from build123d import *

# Parameters (mm, degrees)
F1_DEPTH = 38.1


with BuildPart() as f1:
    # F0 (on Right) → F1 (new body, symmetric)
    with BuildSketch(Plane.YZ):
        with BuildLine():
            ThreePointArc((-6.350009, 50.8), (10.388841, 10.388841), (50.8, -6.350009))
            Line((50.8, -6.350009), (353.615227, -6.350009))
            ThreePointArc((353.615227, -6.350009), (404.926872, 25.635765), (398.802211, 85.789428))
            Line((398.802211, 85.789428), (95.986983, 476.859172))
            ThreePointArc((95.986983, 476.859172), (32.310989, 495.946356), (-6.350009, 441.869744))
            Line((-6.350009, 441.869744), (-6.350009, 50.8))
        make_face()
        with BuildLine():
            Line((0, 50.8), (0, 441.869744))
            ThreePointArc((0, 441.869744), (34.365327, 489.937836), (90.966201, 472.971453))
            Line((90.966201, 472.971453), (393.781428, 81.901709))
            ThreePointArc((393.781428, 81.901709), (399.22557, 28.431795), (353.615227, 0))
            Line((353.615227, 0), (50.8, 0))
            ThreePointArc((50.8, 0), (14.878976, 14.878976), (0, 50.8))
        make_face(mode=Mode.SUBTRACT)
    extrude(amount=F1_DEPTH, both=True)


solid = f1.part
For this review, take the finished solid that the model builds, in its own axes (mm). A direction names the side the tool comes from. Round coordinates to 2 decimals unless told otherwise and drop trailing zeros. Loops run counter-clockwise (first coordinate to the right, second up) from the corner with the lowest first, then second, coordinate; pieces in that order, holes last. Notation, with made-up numbers: (37.25, 83.5) - (42.25, 83.5) arc R15 ccw to (42.25, 93.5) - close; hole circle Ø10 at (-24.75, 61). An arc over 180 degrees is marked (long way). Use one line per item in the form item = value.
Item 1: Consider section B-B on x = -13.5. Write out the cut boundary in (y, z).
Answers:
outline = (-6.35, 50.8) arc R57.15 ccw to (50.8, -6.35) - (353.62, -6.35) arc R57.15 ccw to (398.8, 85.79) - (95.99, 476.86) arc R57.15 ccw to (-6.35, 441.87) - close; hole (0, 50.8) arc R50.8 ccw to (50.8, 0) - (353.62, 0) arc R50.8 ccw to (393.78, 81.9) - (90.97, 472.97) arc R50.8 ccw to (0, 441.87) - close
Item 2: Mouldability with a two-part tool opening along Y and no side actions: class faces 1 (the cylindrical face through (0.533, 33.532, 489.645)), 2 (the cylindrical face through (0.53, 33.25, 496.26)), 3 (the flat face through (38.1, 186, 360)) as +Y half, -Y half, draft (parallel to the pull), parting line (faces both ways), or undercut.
Answers:
face_1 = undercut
face_2 = parting line
face_3 = draft
Item 3: Consider section C-C on z = 343.5. Write out the cut boundary in (x, y).
Answers:
outline = (-38.1, -6.35) - (38.1, -6.35) - (38.1, 0) - (-38.1, 0) - close; (-38.1, 191.22) - (38.1, 191.22) - (38.1, 199.25) - (-38.1, 199.25) - close
Item 4: For line 1 (Y direction, x = 10.5, z = 329.5); line 2 (Y direction, x = 16, z = 18); line 3 (Z direction, x = -12, y = 268), list the stretches that pass through material, from the lowest coordinate up.
Answers:
line_1 = -6.35 to 0, 202.06 to 210.09
line_2 = 4 to 12.01, 392.41 to 400.42
line_3 = -6.35 to 0, 244.34 to 254.71
Item 5: Consider section A-A on y = 164. Write out the cut boundary in (x, z), then the cut area to 3 significant figures.
Answers:
outline = (-38.1, -6.35) - (38.1, -6.35) - (38.1, 0) - (-38.1, 0) - close; (-38.1, 378.65) - (38.1, 378.65) - (38.1, 389.02) - (-38.1, 389.02) - close
area = 1,270 mm^2
Item 6: Clearance check with flat-ended pins moving along their axes: P1, Ø8, axis at x = -16, y = 290.5, coming from the +Z side; P2, Ø6, axis at x = -6, y = 143.5, coming from the +Z side; P3, Ø1.5, axis at x = 15.5, z = 108, coming from the +Y side. State where each tip first meets the part, or that it passes through.
Answers:
P1 = 230.82
P2 = 419.37
P3 = 382.18
Item 7: Tool access review of faces 4 (the flat face through (1, -6.35, 249)), 5 (the cylindrical face through (0.533, 15.276, 14.486)): name each direction out of +Z, -Z, +X, -X, +Y, -Y from which nothing blocks a thin tool from reaching the whole face with its end or side.
Answers:
face_4 = +Z, -Z, +X, -X, -Y
face_5 = +X, -X
